Check sheet for the modelled part. Datum: model origin and axes. Units: mm. Round coordinates to 2 decimals unless told otherwise and drop trailing zeros. Loops run counter-clockwise (first coordinate to the right, second up) from the corner with the lowest first, then second, coordinate; pieces in that order, holes last. Notation, with made-up numbers: (-30.75, -31) - (-6.75, -31) arc R19 cw to (-6.75, -3) - close; hole circle Ø10 at (88, 70.25). An arc over 180 degrees is marked (long way). Return JSON: item names as keys, results as strings.
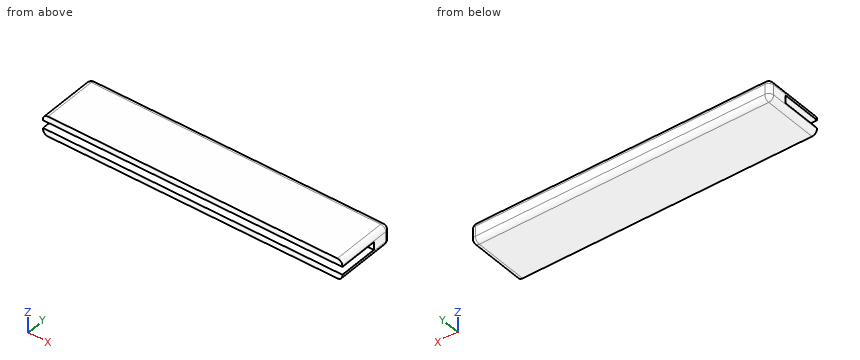
from build123d import *

# Parameters (mm, degrees)
F0_W     = 76.2
F0_H     = 5.08
F1_DEPTH = 15.24
F2_W     = 76.2
F2_H     = 1.9812
F3_DEPTH = 10.16
F4_R     = 1.27


with BuildPart() as f1:
    # F0 (on Front) → F1 (new body)
    with BuildSketch(Plane.XZ):
        with Locations((0, 2.54)):
            Rectangle(F0_W, F0_H)
    extrude(amount=F1_DEPTH)

    # F2 (on face) → F3 (cut)
    with BuildSketch(Plane.XZ.offset(15.24)):
        with Locations((0, 2.54)):
            Rectangle(F2_W, F2_H)
    extrude(amount=-F3_DEPTH, mode=Mode.SUBTRACT)

    # F4
    f4_edges = [f1.edges().sort_by_distance(p)[0] for p in [
        (0, 0, 5.08),
        (0, 0, 0),
        (-38.1, 0, 2.54),
        (38.1, 0, 2.54),
        (38.1, -7.62, 5.08),
        (38.1, -7.62, 0),
        (-38.1, -7.62, 5.08),
        (-38.1, -7.62, 0),
    ]]
    fillet(f4_edges, radius=F4_R)


solid = f1.part
Q1. Scan lines: probe 1 along Z at (x, y) = (13.5, -6.5); probe 2 along Y at (x, z) = (17, 2); probe 3 along Y at (x, z) = (-28.5, 4.85). Record each from-to range of solid material in increasing order. Write a range as [from, to].
Answer key:
{"probe 1": "z = [0, 1.55], [3.53, 5.08]", "probe 2": "y = [-5.08, 0]", "probe 3": "y = [-15.24, -0.54]"}
Q2. Sectioned sample at B-B (x = -17). Enter the section's corners in (y, z), plus the area to 3 significant figures.
Answer key:
{"outline": "(-15.24, 0) - (-1.27, 0) arc R1.27 ccw to (0, 1.27) - (0, 3.81) arc R1.27 ccw to (-1.27, 5.08) - (-15.24, 5.08) - (-15.24, 3.53) - (-5.08, 3.53) - (-5.08, 1.55) - (-15.24, 1.55) - close", "area": "56.6 mm²"}
Q3. Sectioned sample at A-A (y = -5.75). Enter the section's corners in (x, z).
Answer key:
{"outline": "(-38.1, 1.27) arc R1.27 ccw to (-36.83, 0) - (36.83, 0) arc R1.27 ccw to (38.1, 1.27) - (38.1, 1.55) - (-38.1, 1.55) - close; (-38.1, 3.53) - (38.1, 3.53) - (38.1, 3.81) arc R1.27 ccw to (36.83, 5.08) - (-36.83, 5.08) arc R1.27 ccw to (-38.1, 3.81) - close"}
